from build123d import *

# Parameters (mm, degrees)
SKETCH3_R           = 40
BOSS_EXTRUDE1_DEPTH = 6
SKETCH4_R           = 2.1
CUT_EXTRUDE1_DEPTH  = 57.885850613
SKETCH5_R           = 5
CUT_EXTRUDE2_DEPTH  = 1.5
MOVE_FACE1_BY       = 0.4
MOVE_FACE1_2_BY     = 0.4


with BuildPart() as part:
    # Sketch3 → Boss-Extrude1 (new body)
    with BuildSketch(Plane.XY):
        Circle(SKETCH3_R)
    extrude(amount=BOSS_EXTRUDE1_DEPTH)

    # Sketch4 → Cut-Extrude1 (cut, through all)
    with BuildSketch(Plane.XY.offset(6)):
        with Locations((-17.5, -8)):
            Circle(SKETCH4_R)
        with Locations((17.5, -8)):
            Circle(SKETCH4_R)
    extrude(amount=-CUT_EXTRUDE1_DEPTH, mode=Mode.SUBTRACT)

    # Sketch5 → Cut-Extrude2 (cut)
    with BuildSketch(Plane(origin=(0, 0, 0), x_dir=(-1, 0, 0), z_dir=(0, 0, -1))):
        with Locations((-17.5, -8)):
            Circle(SKETCH5_R)
        with Locations((17.5, -8)):
            Circle(SKETCH5_R)
    extrude(amount=-CUT_EXTRUDE2_DEPTH, mode=Mode.SUBTRACT)

    # Move Face1: a curved face moved inward by 0.4
    add(Solid.thicken(part.faces().sort_by_distance((-19.6, -8, 3.75))[0], -MOVE_FACE1_BY), mode=Mode.SUBTRACT)

    # Move Face1 2: a curved face moved inward by 0.4
    add(Solid.thicken(part.faces().sort_by_distance((15.4, -8, 3.75))[0], -MOVE_FACE1_2_BY), mode=Mode.SUBTRACT)


solid = part.part
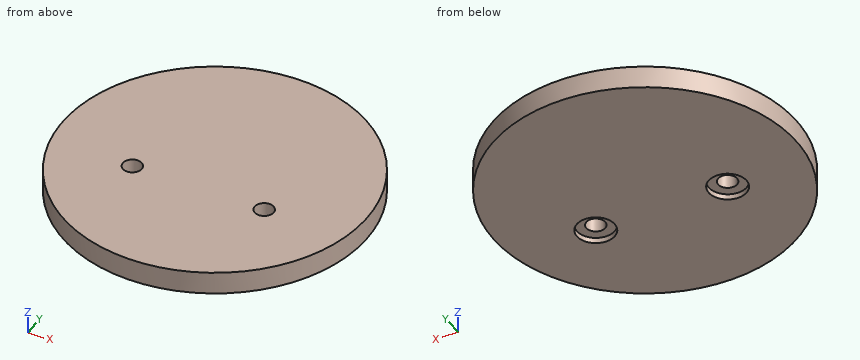
Geometry: final body of the model. Coordinates: model frame, mm. Round coordinates to 2 decimals unless told otherwise and drop trailing zeros. Order: outer loops, then holes, each group sorted by start corner. A loop starts at its lowest first (then second) coordinate and runs counter-clockwise, first axis right, second up.
Q1. Pin query (flat end, axial travel): pin 1 (2 mm diameter, centred on x = -19, z = 3.5, fed in from -Y); pin 2 (8 mm diameter, centred on x = -17.5, y = -8, fed in from -Z). Return the tip coordinate at first contact, or that it passes through.
Result sheet:
pin 1: stops at y = -35.72
pin 2: stops at z = 1.5
Q2. Material intervals for probe 1 along Z at (x, y) = (20, -11); probe 2 along Y at (x, z) = (17.5, 2.9); probe 3 along X at (y, z) = (-30, 3.6), sorted ascending.
Result sheet:
probe 1: z = 1.5 to 6
probe 2: y = -35.97 to -10.5, -5.5 to 35.97
probe 3: x = -26.46 to 26.46
Q3. Section B-B, the plane y = -9. Output: boundary loops of the cut face in (x, z).
Result sheet:
outline: (-38.97, 0) - (-22.4, 0) - (-22.4, 1.5) - (-19.79, 1.5) - (-19.79, 6) - (-38.97, 6) - close; (-15.21, 1.5) - (-12.6, 1.5) - (-12.6, 0) - (12.6, 0) - (12.6, 1.5) - (15.21, 1.5) - (15.21, 6) - (-15.21, 6) - close; (19.79, 1.5) - (22.4, 1.5) - (22.4, 0) - (38.97, 0) - (38.97, 6) - (19.79, 6) - close
Q4. Section C-C, the plane z = 2.95. Output: boundary loops of the cut face in (x, y), and give its area (3 significant figures).
Result sheet:
outline: circle Ø80 at (0, 0); hole circle Ø5 at (-17.5, -8); hole circle Ø5 at (17.5, -8)
area: 4,990 mm2
Q5. Section A-A, the plane x = -16.5. Output: boundary loops of the cut face in (y, z).
Result sheet:
outline: (-36.44, 0) - (-12.9, 0) - (-12.9, 1.5) - (-10.29, 1.5) - (-10.29, 6) - (-36.44, 6) - close; (-5.71, 1.5) - (-3.1, 1.5) - (-3.1, 0) - (36.44, 0) - (36.44, 6) - (-5.71, 6) - close
Q6. Section D-D, the plane x = 17.5. Output: boundary loops of the cut face in (y, z).
Result sheet:
outline: (-35.97, 0) - (-13, 0) - (-13, 1.5) - (-10.5, 1.5) - (-10.5, 6) - (-35.97, 6) - close; (-5.5, 1.5) - (-3, 1.5) - (-3, 0) - (35.97, 0) - (35.97, 6) - (-5.5, 6) - close
